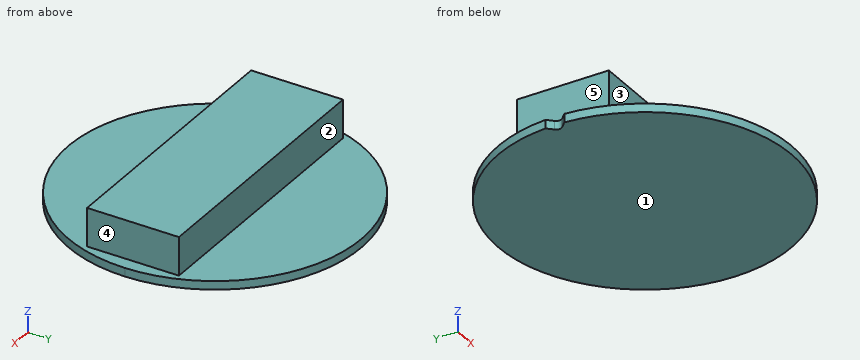
```python
from build123d import *

# Parameters (mm, degrees)
SKETCH_1_R          = 27.5
EXTRUDE_1_DEPTH     = 1.6
SKETCH_2_W          = 50
SKETCH_2_H          = 17.24
EXTRUDE_2_DEPTH     = 7.2
CUT_EXTRUDE_1_DEPTH = 40.551738268


with BuildPart() as part:
    # 草图1 → 凸台-拉伸1 (new body)
    with BuildSketch(Plane.XY):
        Circle(SKETCH_1_R)
    extrude(amount=EXTRUDE_1_DEPTH)

    # 草图2 → 凸台-拉伸2 (add)
    with BuildSketch(Plane.XY.offset(1.6)):
        Rectangle(SKETCH_2_W, SKETCH_2_H)
    extrude(amount=EXTRUDE_2_DEPTH)

    # 草图3 → 切除-拉伸1 (cut, through all)
    with BuildSketch(Plane.XY.offset(1.6)):
        with BuildLine():
            Line((-27.443123, 1.767766953), (-26.382462828, 0.707106781))
            ThreePointArc((-26.382462828, 0.707106781), (-26.08956961, 0), (-26.382462828, -0.707106781))
            Line((-26.382462828, -0.707106781), (-27.443123, -1.767766953))
            ThreePointArc((-27.443123, -1.767766953), (-27.5, 0), (-27.443123, 1.767766953))
        make_face()
    extrude(amount=-CUT_EXTRUDE_1_DEPTH, mode=Mode.SUBTRACT)


solid = part.part
```
Work out the finished part from the listing and answer in its coordinate system (mm). Face numbers are marked on the shaded views. A direction names the side the tool comes from. Give positions to 0.01 mm unless a question says otherwise; leave off trailing zeros. Write each loop counter-clockwise with the first axis right and the second up, starting at its lowest first coordinate (ties: lowest second). Pieces come first, ordered by that corner, then holes. Notation, with made-up numbers: (60.25, 73.25) -> (109.25, 73.25) arc R21 ccw to (109.25, 90.25) -> close; hole circle Ø7 at (-9, 68). An arc over 180 degrees is marked (long way). Write each question's results on one line, items separated by ' | '.
1. A tool of negligible diameter and unlimited length cuts with its end or side. For the marked faces 1, 2, 3, 4 and 5, from which of +Z, -Z, +X, -X, +Y, -Y can it reach the whole face along a straight path? Write none if from no direction.
Data:
face 1: -Z, +X, -X, +Y, -Y | face 2: +Z, +X, -X, +Y | face 3: +Z, +X, -X, -Y | face 4: +Z, +X, +Y, -Y | face 5: +Z, -X, +Y, -Y
2. Find section D-D on x = 0. Determine the outline of the cut face in (y, z).
Data:
outline: (-27.5, 0) -> (27.5, 0) -> (27.5, 1.6) -> (8.62, 1.6) -> (8.62, 8.8) -> (-8.62, 8.8) -> (-8.62, 1.6) -> (-27.5, 1.6) -> close
3. Each of these flat-tipped pins is pushed along its axis until it touches: pin 1 Ø3.5 at (y, z) = (2, 4) entering from -X; pin 2 Ø2 at (x, z) = (-21, 4) entering from +Y; pin 3 Ø5 at (y, z) = (-6.5, 2.5) entering from +X. Where does it stop, or does it pass through?
Data:
pin 1: x = -25 | pin 2: y = 8.62 | pin 3: x = 27.18
4. Straight lines are drawn through the part: L1, parallel to Y at x = -21, z = 5.25; L2, parallel to Z at x = 3.5, y = -9; L3, parallel to X at y = -3.5, z = 7. For each, find the intervals that lie inside material, in ascending order.
Data:
L1: -8.62 to 8.62 | L2: 0 to 1.6 | L3: -25 to 25
5. Find section A-A on x = -18.5. Determine the outline of the cut face in (y, z).
Data:
outline: (-20.35, 0) -> (20.35, 0) -> (20.35, 1.6) -> (8.62, 1.6) -> (8.62, 8.8) -> (-8.62, 8.8) -> (-8.62, 1.6) -> (-20.35, 1.6) -> close
6. Find section B-B on z = 5.75. Determine the outline of the cut face in (x, y).
Data:
outline: (-25, -8.62) -> (25, -8.62) -> (25, 8.62) -> (-25, 8.62) -> close
7. Find section C-C on y = -13.5. Determine the outline of the cut face in (x, z), and give its area (3 significant figures).
Data:
outline: (-23.96, 0) -> (23.96, 0) -> (23.96, 1.6) -> (-23.96, 1.6) -> close | area: 76.7 mm^2
